```python
from build123d import *

# Parameters (mm, degrees)
SKETCH1_R           = 2.5
BOSS_EXTRUDE1_DEPTH = 3


with BuildPart() as part:
    # Sketch1 → Boss-Extrude1 (new body)
    # profile 1 of 4: a face of its own
    with BuildSketch(Plane.XY):
        with BuildLine():
            Line((29.001181793, 36.666122725), (9.001181793, 36.666122725))
            Line((9.001181793, 36.666122725), (9.001181793, 34.166122725))
            ThreePointArc((9.001181793, 34.166122725), (10.768948746, 33.433889678), (11.501181793, 31.666122725))
            Line((11.501181793, 31.666122725), (14.001181793, 31.666122725))
            Line((14.001181793, 31.666122725), (14.001181793, 26.666122725))
            Line((14.001181793, 26.666122725), (29.001181793, 26.666122725))
            ThreePointArc((29.001181793, 26.666122725), (34.001181793, 31.666122725), (29.001181793, 36.666122725))
        make_face()
        with Locations((29.001181793, 31.666122725)):
            Circle(SKETCH1_R, mode=Mode.SUBTRACT)
    # profile 2 of 4: a face of its own
    with BuildSketch(Plane.XY):
        with BuildLine():
            Line((4.001181793, 31.666122725), (4.001181793, 11.666122725))
            ThreePointArc((4.001181793, 11.666122725), (9.001181793, 6.666122725), (14.001181793, 11.666122725))
            Line((14.001181793, 11.666122725), (14.001181793, 26.666122725))
            Line((14.001181793, 26.666122725), (9.001181793, 26.666122725))
            Line((9.001181793, 26.666122725), (9.001181793, 29.166122725))
            ThreePointArc((9.001181793, 29.166122725), (7.23341484, 29.898355772), (6.501181793, 31.666122725))
            Line((6.501181793, 31.666122725), (4.001181793, 31.666122725))
        make_face()
        with Locations((9.001181793, 11.666122725)):
            Circle(SKETCH1_R, mode=Mode.SUBTRACT)
    # profile 3 of 4: a face of its own
    with BuildSketch(Plane.XY):
        with BuildLine():
            Line((9.001181793, 26.666122725), (14.001181793, 26.666122725))
            Line((14.001181793, 26.666122725), (14.001181793, 31.666122725))
            Line((14.001181793, 31.666122725), (11.501181793, 31.666122725))
            ThreePointArc((11.501181793, 31.666122725), (10.768948746, 29.898355772), (9.001181793, 29.166122725))
            Line((9.001181793, 29.166122725), (9.001181793, 26.666122725))
        make_face()
    # profile 4 of 4: a face of its own
    with BuildSketch(Plane.XY):
        with BuildLine():
            ThreePointArc((9.001181793, 36.666122725), (5.465647887, 35.201656631), (4.001181793, 31.666122725))
            Line((4.001181793, 31.666122725), (6.501181793, 31.666122725))
            ThreePointArc((6.501181793, 31.666122725), (7.23341484, 33.433889678), (9.001181793, 34.166122725))
            Line((9.001181793, 34.166122725), (9.001181793, 36.666122725))
        make_face()
    extrude(amount=BOSS_EXTRUDE1_DEPTH)


solid = part.part
```
Read the model definition and answer for the solid it produces. Units are mm, in the model's axes. A direction names the side the tool comes from. Coordinates: 2 decimals unless noted, no trailing zeros. Write each loop counter-clockwise with the first axis right and the second up, starting at its lowest first coordinate (ties: lowest second). Pieces come first, ordered by that corner, then holes. Notation, with made-up numbers: (53.5, 56.5) -> (66.5, 56.5) arc R35 ccw to (66.5, 91.5) -> close; hole circle Ø3 at (19, -40). An arc over 180 degrees is marked (long way). Return JSON: item names as keys, results as strings.
1. A cutting plane is placed at C-C (y = 21.75). Determine the outline of the cut face in (x, z), and give its area (3 significant figures).
Found:
{"outline": "(4, 0) -> (14, 0) -> (14, 3) -> (4, 3) -> close", "area": "30.0 mm2"}
2. Find the intervals of material crossed by line 1 along Y through (x, z) = (8.75, 0.3); line 2 along X through (y, z) = (31, 2.7); line 3 along X through (y, z) = (33.25, 2.1), in increasing order. Write a range as from..to.
Found:
{"line 1": "6.67..9.18, 14.15..29.18, 34.15..36.66", "line 2": "4..6.59, 11.41..26.59, 31.41..33.96", "line 3": "4.26..7.07, 10.94..27.07, 30.94..33.74"}
3. A cutting plane is placed at B-B (x = 22.5). Determine the outline of the cut face in (y, z).
Found:
{"outline": "(26.67, 0) -> (36.67, 0) -> (36.67, 3) -> (26.67, 3) -> close"}
4. A cutting plane is placed at A-A (z = 0.5). Determine the outline of the cut face in (x, y), and give its area (3 significant figures).
Found:
{"outline": "(4, 11.67) arc R5 ccw to (14, 11.67) -> (14, 26.67) -> (29, 26.67) arc R5 ccw to (29, 36.67) -> (9, 36.67) arc R5 ccw to (4, 31.67) -> close; hole circle Ø5 at (9, 11.67); hole circle Ø5 at (9, 31.67); hole circle Ø5 at (29, 31.67)", "area": "414 mm2"}
5. Each of these flat-tipped pins is pushed along its axis until it touches: P1, Ø4, axis at x = 29, y = 31.67, coming from the -Z side; P2, Ø1.5, axis at y = 16, z = 1.5, coming from the +X side. Where does it stop, or does it pass through?
Found:
{"P1": "through", "P2": "x = 14"}
6. A tool of negligible diameter and unlimited length cuts with its end or side. For faces 1 (the face through (8.891, 6.667, 1.479)), 2 (the face through (21, 26.666, 1)), from which of +Z, -Z, +X, -X, +Y, -Y can it reach the whole face along a straight path? Write none if from no direction.
Found:
{"face 1": "+Z, -Z, -Y", "face 2": "+Z, -Z, +X, -Y"}
